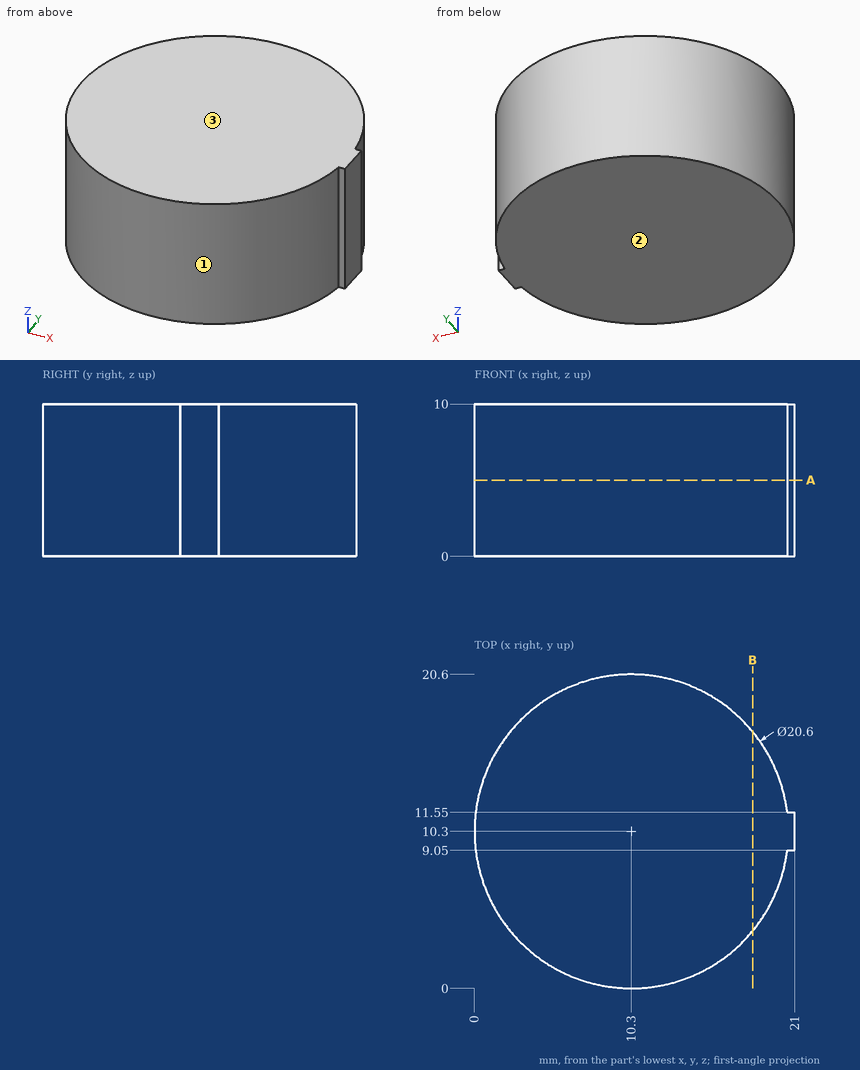
Print and shaded views of the part. All mm, measured from the part's lowest x, y and z. Coordinates: 2 decimals unless noted, no trailing zeros. Loops run counter-clockwise (first coordinate to the right, second up) from the corner with the lowest first, then second, coordinate; pieces in that order, holes last. Notation, with made-up numbers: M 24.25,87.5 L 77.25,87.5 A33 ccw 77.25,125.5 Z; hole C 12.5,17.5 d7. An arc over 180 degrees is marked long. Use a Markdown table: item, result. Add a question column.
Q1. Cut at A-A (z = 5). Write the cut outline in (x, y), and give its area (3 significant figures).
Q2. Probe L1, parallel to X at y = 10, z = 1; L2, parallel to Y at x = 10, z = 5.75; L3, parallel to Y at x = 8, z = 3.5. List the from-to ranges inside material, lowest first.
Q3. Cut at B-B (x = 18.25). Write the cut outline in (y, z), and give its area (3 significant figures).
Q4. Mould opens along Z. For the marked faces 1, 2 and 3 say: +Z half, -Z half, draft (parallel to the pull), parting line (faces both ways), or undercut.
Q5. Pin check, flat tips, straight feed: P1, Ø1.5, axis at y = 14.5, z = 5.5, coming from the +X side (3 decimals); P2, Ø2, axis at x = 14, z = 8.5, coming from the -Y side; P3, Ø4, axis at x = 5, z = 1.5, coming from the +Y side. Stop position of each tip, or through.
Worked out:
| question | item | result |
|---|---|---|
| 1 | outline | M 20.52,9.05 L 21,9.05 L 21,11.55 L 20.52,11.55 A10.3 ccw long Z |
| 1 | area | 334 mm2 |
| 2 | L1 | x = 0 to 21 |
| 2 | L2 | y = 0 to 20.6 |
| 2 | L3 | y = 0.26 to 20.34 |
| 3 | outline | M 3.75,0 L 16.85,0 L 16.85,10 L 3.75,10 Z |
| 3 | area | 131 mm2 |
| 4 | face 1 | draft |
| 4 | face 2 | -Z half |
| 4 | face 3 | +Z half |
| 5 | P1 | stops at x = 20.005 |
| 5 | P2 | stops at y = 0.36 |
| 5 | P3 | stops at y = 20.06 |
